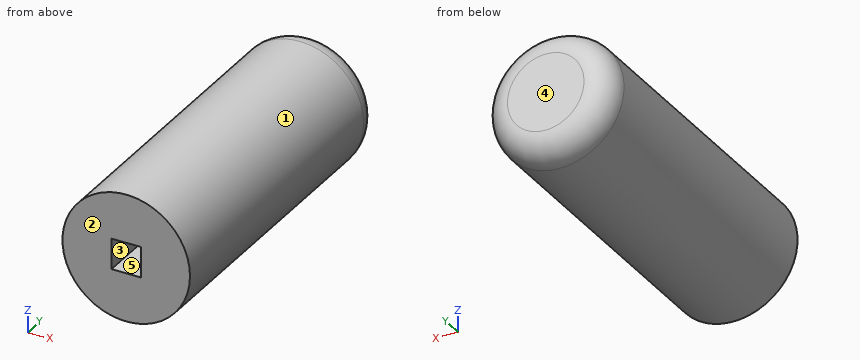
```python
from build123d import *

# Parameters (mm, degrees)
SKETCH2_R           = 2.5
SKETCH2_W           = 1.15
SKETCH2_H           = 1.2
BOSS_EXTRUDE1_DEPTH = 6.5
FILLET1_R           = 1
SKETCH3_W           = 1.15
SKETCH3_H           = 1.2
BOSS_EXTRUDE5_DEPTH = 1


with BuildPart() as part:
    # Sketch2 → Boss-Extrude1 (new body, symmetric)
    with BuildSketch(Plane(origin=(0, 0, 0), x_dir=(1, 0, 0), z_dir=(0, 1, 0))):
        Circle(SKETCH2_R)
        Rectangle(SKETCH2_W, SKETCH2_H, mode=Mode.SUBTRACT)
    extrude(amount=BOSS_EXTRUDE1_DEPTH, both=True)

    # Fillet1
    fillet1_edges = [part.edges().sort_by_distance(p)[0] for p in [
        (-2.5, 6.5, 0),
    ]]
    fillet(fillet1_edges, radius=FILLET1_R)

    # Sketch3 → Boss-Extrude5 (add)
    with BuildSketch(Plane(origin=(0, 6.5, 0), x_dir=(1, 0, 0), z_dir=(0, 1, 0))):
        Rectangle(SKETCH3_W, SKETCH3_H)
    extrude(amount=-BOSS_EXTRUDE5_DEPTH)


solid = part.part
```
Here's how the part is built. I have some questions about the finished solid (model axes, mm). Face numbers are marked on the shaded views. A direction names the side the tool comes from. Round coordinates to 2 decimals unless told otherwise and drop trailing zeros. Order: outer loops, then holes, each group sorted by start corner. A loop starts at its lowest first (then second) coordinate and runs counter-clockwise, first axis right, second up. Notation, with made-up numbers: M 85,58 L 112,58 A15 cw 112,68 Z; hole C 85,54.5 d9. An arc over 180 degrees is marked long. One line per question, with ' | ' between items.
1) I want a section at C-C, the plane z = 0. Write out the boundary of the cut face in (x, y) (3 decimals), then the cut area to 3 significant figures.
Working result:
outline: M -2.5,-6.5 L -0.575,-6.5 L -0.575,5.5 L 0.575,5.5 L 0.575,-6.5 L 2.5,-6.5 L 2.5,5.5 A1 ccw 1.5,6.5 L -1.5,6.5 A1 ccw -2.5,5.5 Z | area: 50.8 mm²
2) I want a section at A-A, the plane x = 0. Write out the boundary of the cut face in (y, z).
Working result:
outline: M -6.5,-2.5 L 5.5,-2.5 A1 ccw 6.5,-1.5 L 6.5,1.5 A1 ccw 5.5,2.5 L -6.5,2.5 L -6.5,0.6 L 5.5,0.6 L 5.5,-0.6 L -6.5,-0.6 Z
3) I need wall thicknesses on line 1 along Z through (x, y) = (-0.05, -1.5); line 2 along X through (y, z) = (-4.25, 0) (3 decimals); line 3 along Z through (x, y) = (0.5, 1.5). Which ranges of each line are inside material? Lowest first, please.
Working result:
line 1: -2.5 to -0.6, 0.6 to 2.5 | line 2: -2.5 to -0.575, 0.575 to 2.5 | line 3: -2.45 to -0.6, 0.6 to 2.45
4) For the marked faces 4 and 5, which set-ups out of +Z, -Z, +X, -X, +Y, -Y let a thin tool reach every point of the face, with its end or its side?
Working result:
face 4: +Z, -Z, +X, -X, +Y | face 5: -Y
5) If we mould it in two halves opening along Z, with no side actions, what happens to the marked faces 1, 2 and 3? For each: +Z half, -Z half, draft (parallel to the pull), parting line (faces both ways), or undercut.
Working result:
face 1: parting line | face 2: draft | face 3: undercut
6) I want a section at B-B, the plane y = 3.5. Write out the boundary of the cut face in (x, z) (3 decimals).
Working result:
outline: C 0,0 d5; hole M -0.575,-0.6 L 0.575,-0.6 L 0.575,0.6 L -0.575,0.6 Z
7) For pin 1 Ø3 at (y, z) = (-2.5, 2) entering from -X; pin 2 Ø1 at (x, y) = (2, 4) entering from +Z; pin 3 Ø2 at (y, z) = (-1.5, 2) entering from +X, each with a flat end and sliding along its axis, tell me the tip position at first contact or that it passes through.
Working result:
pin 1: x = -2.45 | pin 2: z = 2 | pin 3: x = 2.29
